Source: three-view drawing plus pictorial views. Frame: mm from the lowest corner of the part. Coordinates: 2 decimals unless noted, no trailing zeros. Write each loop counter-clockwise with the first axis right and the second up, starting at its lowest first coordinate (ties: lowest second). Pieces come first, ordered by that corner, then holes. Notation, with made-up numbers: (37, 81) -> (44, 81) arc R32 ccw to (44, 110) -> close; hole circle Ø8 at (-14.75, -32). An arc over 180 degrees is marked (long way). Write item = value, one per line.
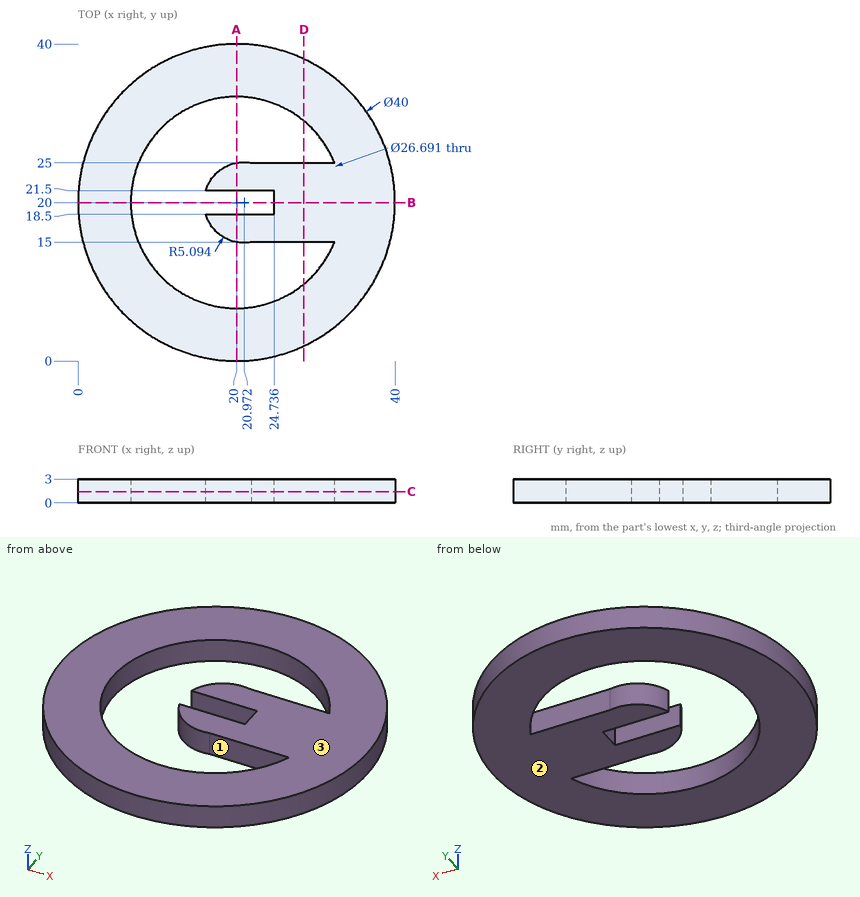
1) Material intervals for probe 1 along Y at (x, z) = (20, 0.6) (1 decimal); probe 2 along Y at (x, z) = (28, 0.3); probe 3 along Y at (x, z) = (12, 0.65), sorted ascending. Write a range as [from, to].
Answer block:
probe_1 = [0, 6.7], [15, 18.5], [21.5, 25], [33.3, 40]
probe_2 = [1.67, 9.32], [15, 25], [30.68, 38.33]
probe_3 = [1.67, 9.32], [30.68, 38.33]
2) Pull-direction query (Z, two-part tool) for the marked faces 1, 2 and 3; classes: +Z half, -Z half, draft (parallel to the pull), parting line (faces both ways), or undercut.
Answer block:
face_1 = draft
face_2 = -Z half
face_3 = +Z half
3) First-contact query: pin 1 Ø1 at (x, y) = (4.5, 5) entering from -Z; pin 2 Ø1.5 at (y, z) = (18, 0.5) entering from +X; pin 3 Ø0.9 at (x, z) = (25, 2) entering from -Y (1 decimal); pin 4 Ø1.5 at (x, z) = (27, 1) entering from +Y. Flat tips, straight axial feed; report the tip coordinate or a pass-through.
Answer block:
pin_1 = through
pin_2 = 39.96
pin_3 = 0.5
pin_4 = 39
4) Cut plane C-C, the plane z = 1.4. Output: boundary loops of the cut face in (x, y) (1 decimal), and give its area (3 significant figures).
Answer block:
outline = circle Ø40 at (20, 20); hole (16.1, 18.5) -> (24.7, 18.5) -> (24.7, 21.5) -> (16.1, 21.5) arc R5.1 cw to (21.9, 25) -> (32.4, 25) arc R13.3 ccw (long way) to (32.4, 15) -> (21.9, 15) arc R5.1 cw to start
area = 832 mm2
5) Cut plane D-D, the plane x = 28.5. Output: boundary loops of the cut face in (y, z).
Answer block:
outline = (1.9, 0) -> (9.71, 0) -> (9.71, 3) -> (1.9, 3) -> close; (15, 0) -> (25, 0) -> (25, 3) -> (15, 3) -> close; (30.29, 0) -> (38.1, 0) -> (38.1, 3) -> (30.29, 3) -> close
6) Cut plane B-B, the plane y = 20. Output: boundary loops of the cut face in (x, z) (1 decimal).
Answer block:
outline = (0, 0) -> (6.7, 0) -> (6.7, 3) -> (0, 3) -> close; (24.7, 0) -> (40, 0) -> (40, 3) -> (24.7, 3) -> close
7) Cut plane A-A, the plane x = 20. Output: boundary loops of the cut face in (y, z) (1 decimal).
Answer block:
outline = (0, 0) -> (6.7, 0) -> (6.7, 3) -> (0, 3) -> close; (15, 0) -> (18.5, 0) -> (18.5, 3) -> (15, 3) -> close; (21.5, 0) -> (25, 0) -> (25, 3) -> (21.5, 3) -> close; (33.3, 0) -> (40, 0) -> (40, 3) -> (33.3, 3) -> close
